Source: CAD feature listing. Evaluate the final solid. Frame: model axes, mm. Round coordinates to 2 decimals unless told otherwise and drop trailing zeros. Write each loop counter-clockwise with the first axis right and the second up, starting at its lowest first coordinate (ties: lowest second). Pieces come first, ordered by that corner, then holes. Notation, with made-up numbers: M 82,65 L 101,65 A22 cw 101,98 Z; hole C 86,55 d10. An arc over 180 degrees is marked long. Answer in a Markdown table with one row per item. Add a question column.
Item 1: Cut plane A-A on y = -29.5. Return loops of the section in (x, z).
Item 2: Cut plane B-B on x = 77. Return loops of the section in (y, z), and give its area (3 significant figures).
Item 3: Cut plane C-C on z = 63. Return loops of the section in (x, y).
Item 4: Contact query for flat-ended pins moving along their axis: pin 1 (10 mm diameter, centred on y = -42, z = 8.5, fed in from -X); pin 2 (10 mm diameter, centred on y = -63, z = 45, fed in from -X). Output: stop coordinate, or through.
Item 5: Material intervals for probe 1 along Z at (x, y) = (-12.5, -76); probe 2 along Z at (x, y) = (14, -4); probe 3 along X at (y, z) = (-79.5, 15), sorted ascending.
from build123d import *

# Parameters (mm, degrees)
F0_W     = 177.8
F0_H     = 101.6
F1_DEPTH = 101.6
F3_DEPTH = 101.6


with BuildPart() as f1:
    # F0 (on Front) → F1 (new body)
    with BuildSketch(Plane.XZ):
        with Locations((0, -50.8)):
            Rectangle(F0_W, F0_H)
    extrude(amount=F1_DEPTH)

    # F2 (on face) → F3 (join, through all)
    with BuildSketch(Plane(origin=(0, 0, 0), x_dir=(-1, 0, 0), z_dir=(0, 1, 0))):
        Polygon((-88.9, 0), (88.9, 0), (0, 76.2), align=None)
    extrude(amount=-F3_DEPTH)


solid = f1.part
Results below:
| question | item | result |
|---|---|---|
| 1 | outline | M -88.9,-101.6 L 88.9,-101.6 L 88.9,0 L 0,76.2 L -88.9,0 Z |
| 2 | outline | M -101.6,-101.6 L 0,-101.6 L 0,10.2 L -101.6,10.2 Z |
| 2 | area | 11,400 mm2 |
| 3 | outline | M -15.4,-101.6 L 15.4,-101.6 L 15.4,0 L -15.4,0 Z |
| 4 | pin 1 | x = -84.82 |
| 4 | pin 2 | x = -42.23 |
| 5 | probe 1 | -101.6 to 65.49 |
| 5 | probe 2 | -101.6 to 64.2 |
| 5 | probe 3 | -71.4 to 71.4 |
